from build123d import *

# Parameters (mm, degrees)
F1_DEPTH = 25
F2_DEPTH = 5
F3_R     = 5
F5_DEPTH = 1
F6_DEPTH = 5
F8_DEPTH = 1
F9_DEPTH = 5


with BuildPart() as f1:
    # F0 (on Right) → F1 (new body)
    with BuildSketch(Plane.YZ):
        Polygon((-1.9545168432, 38.6489601963), (-33.5964987424, 14.1788767986), (-28.2257758369, -25.4589250511), (-8.406874912, -22.7735635983), (-0.7535947717, -79.2574312341), (4.2011304595, -78.5860908709), (-3.9713255886, -18.2705245759), (3.1545996335, -0.8816359607), (10.2805248557, 16.5072526545), (58.4291094867, 53.742590351), (55.370349062, 57.6978380884), (10.2805248557, 22.8279692467), align=None)
        Polygon((-25.8654488138, -5.6400241263), (-7.3142972833, -13.2422419285), (-9.1963342424, -17.8348428934), (-23.9423909688, -19.8328594567), align=None, mode=Mode.SUBTRACT)
        Polygon((1.5615552233, 8.4168698067), (-1.4719884671, 1.0143288458), (-4.5055321574, -6.3882121151), (-5.26391808, -8.2388473554), (-11.7411414209, -5.5844966263), (-17.2930471416, -3.3093388585), (-23.7702704824, -0.6549881294), (-23.0118845598, 1.1956471108), (-16.944797179, 16.0007290327), (-16.1864112564, 17.851364273), (-9.7091879156, 15.1970135439), (-4.1572821949, 12.9218557761), (2.3199411459, 10.267505047), align=None, mode=Mode.SUBTRACT)
        Polygon((-14.6534166938, 22.50764705), (-2.8510041559, 31.6349520341), (6.2523573083, 19.863500585), (4.1741345282, 14.7921613112), align=None, mode=Mode.SUBTRACT)
        Polygon((-11.7411414209, -5.5844966263), (-10.9827554983, -3.7338613861), (-16.534661219, -1.4587036183), (-17.2930471416, -3.3093388585), align=None)
        Polygon((-10.4675738382, 13.3463783036), (-4.9156681175, 11.0712205358), (-4.1572821949, 12.9218557761), (-9.7091879156, 15.1970135439), align=None)
    extrude(amount=F1_DEPTH)

    # F0 (on Right) → F2 (join)
    with BuildSketch(Plane.YZ):
        Polygon((-5.26391808, -8.2388473554), (-4.5055321574, -6.3882121151), (-10.9827554983, -3.7338613861), (-11.7411414209, -5.5844966263), align=None)
        Polygon((-17.2930471416, -3.3093388585), (-16.534661219, -1.4587036183), (-23.0118845598, 1.1956471108), (-23.7702704824, -0.6549881294), align=None)
        Polygon((-16.944797179, 16.0007290327), (-10.4675738382, 13.3463783036), (-9.7091879156, 15.1970135439), (-16.1864112564, 17.851364273), align=None)
        Polygon((-4.9156681175, 11.0712205358), (1.5615552233, 8.4168698067), (2.3199411459, 10.267505047), (-4.1572821949, 12.9218557761), align=None)
    extrude(amount=F2_DEPTH)

    # F3
    f3_edges = [f1.edges().sort_by_distance(p)[0] for p in [
        (12.5, -33.596499, 14.178877),
    ]]
    fillet(f3_edges, radius=F3_R)

    # F4 (on face) → F5 (join)
    with BuildSketch(Plane(origin=(0, -7.1996627103, 9.3098006026), x_dir=(1, 0, 0), z_dir=(0, -0.6117520849, 0.7910495475))):
        with BuildLine():
            ThreePointArc((14, 56.8474623166), (16, 54.8474623166), (18, 56.8474623166))
            ThreePointArc((18, 56.8474623166), (16, 58.8474623166), (14, 56.8474623166))
        make_face()
        with BuildLine():
            ThreePointArc((14, 44.3474623166), (16, 42.3474623166), (18, 44.3474623166))
            ThreePointArc((18, 44.3474623166), (16, 46.3474623166), (14, 44.3474623166))
        make_face()
        with BuildLine():
            Line((18, 44.3474623166), (18, 56.8474623166))
            ThreePointArc((18, 56.8474623166), (16, 54.8474623166), (14, 56.8474623166))
            Line((14, 56.8474623166), (14, 44.3474623166))
            ThreePointArc((14, 44.3474623166), (16, 46.3474623166), (18, 44.3474623166))
        make_face()
    extrude(amount=F5_DEPTH)

    # F4 (on face) → F6 (cut)
    with BuildSketch(Plane(origin=(0, -7.1996627103, 9.3098006026), x_dir=(1, 0, 0), z_dir=(0, -0.6117520849, 0.7910495475))):
        with BuildLine():
            ThreePointArc((14, 64.8474623166), (16, 62.8474623166), (18, 64.8474623166))
            ThreePointArc((18, 64.8474623166), (16, 66.8474623166), (14, 64.8474623166))
        make_face()
        with BuildLine():
            ThreePointArc((14, 36.3474623166), (16, 34.3474623166), (18, 36.3474623166))
            ThreePointArc((18, 36.3474623166), (16, 38.3474623166), (14, 36.3474623166))
        make_face()
    extrude(amount=-F6_DEPTH, mode=Mode.SUBTRACT)

    # F7 (on face) → F8 (join)
    with BuildSketch(Plane(origin=(0, -11.2853910764, -1.5291137632), x_dir=(1, 0, 0), z_dir=(0, -0.9909450462, -0.1342680726))):
        with BuildLine():
            ThreePointArc((14, -43.6885751417), (16, -45.6885751417), (18, -43.6885751417))
            ThreePointArc((18, -43.6885751417), (16, -41.6885751417), (14, -43.6885751417))
        make_face()
        with BuildLine():
            Line((18, -56.1885751417), (18, -43.6885751417))
            ThreePointArc((18, -43.6885751417), (16, -45.6885751417), (14, -43.6885751417))
            Line((14, -43.6885751417), (14, -56.1885751417))
            ThreePointArc((14, -56.1885751417), (16, -54.1885751417), (18, -56.1885751417))
        make_face()
        with BuildLine():
            ThreePointArc((14, -56.1885751417), (16, -58.1885751417), (18, -56.1885751417))
            ThreePointArc((18, -56.1885751417), (16, -54.1885751417), (14, -56.1885751417))
        make_face()
    extrude(amount=F8_DEPTH)

    # F7 (on face) → F9 (cut)
    with BuildSketch(Plane(origin=(0, -11.2853910764, -1.5291137632), x_dir=(1, 0, 0), z_dir=(0, -0.9909450462, -0.1342680726))):
        with BuildLine():
            ThreePointArc((14, -35.6885751417), (16, -37.6885751417), (18, -35.6885751417))
            ThreePointArc((18, -35.6885751417), (16, -33.6885751417), (14, -35.6885751417))
        make_face()
        with BuildLine():
            ThreePointArc((14, -64.1885751417), (16, -66.1885751417), (18, -64.1885751417))
            ThreePointArc((18, -64.1885751417), (16, -62.1885751417), (14, -64.1885751417))
        make_face()
    extrude(amount=-F9_DEPTH, mode=Mode.SUBTRACT)


solid = f1.part
The model under review builds one solid part; all positions refer to its coordinate system, in mm. A direction names the side the tool comes from. Round coordinates to 2 decimals unless told otherwise and drop trailing zeros. Order: outer loops, then holes, each group sorted by start corner. A loop starts at its lowest first (then second) coordinate and runs counter-clockwise, first axis right, second up. Notation, with made-up numbers: (86, 6) -> (135, 6) arc R34 cw to (135, 44) -> close; hole circle Ø4 at (-11, -16.75). An arc over 180 degrees is marked (long way). Use CSV: the item, a comma, the result in double quotes. Start each with the question number.
(1) Consider section A-A on y = -19. Write out the cut boundary in (x, z), and give its area (3 significant figures).
(2) Consider section B-B on x = 20.75. State how many separate pieces and enclosed holes the cut face has, and give its area (3 significant figures).
(3) Mouldability with a two-part tool opening along Z and no side actions: class faces 1 (the face through (0, -1, 0)), 2 (the face through (14, -4.1, -36.5)), 3 (the face through (12.325, 4.249, 30.628)) as pulls with the +Z half, pulls with the -Z half, needs draft (parallel to the pull), parting line crosses it, or undercut.
(4) Wall thickness on probe 1 along Z at (x, y) = (5.75, -9); probe 2 along Z at (x, y) = (10.5, -14.5); probe 3 along Y at (x, z) = (16.25, 30.5): over which ranges is each line inside the solid? List them lowest first. Write a range as from..to.
(5) Tool access review of faces 4 (the face through (18, 32.5, 40.6)), 5 (the face through (18, -5, -51)), 6 (the face through (12.325, -18.455, -24.135)), 7 (the face through (14.86, -20.49, -2)): name each direction out of +Z, -Z, +X, -X, +Y, -Y from which nothing blocks a thin tool from reaching the whole face with its end or side.
(6) Consider section C-C on y = 34. Write out the cut boundary in (x, z).
(7) Insertion check: pin 1 (5 mm diameter, centred on x = 18, z = -26.5, fed in from +Y); pin 2 (3.5 mm diameter, centred on y = -7, z = -5, fed in from +X); pin 3 (8 mm diameter, centred on x = 15, z = -38, fed in from +Y). Each pin has a flat end and moves straight along its axis. Give the tip position at first contact, or say it passes through.
(8) Consider section D-D on y = 18.5. Write out the cut boundary in (x, z), and give its area (3 significant figures).
Responses:
1,outline,"(0, -24.21) -> (25, -24.21) -> (25, -19.16) -> (0, -19.16) -> close; (0, -8.45) -> (25, -8.45) -> (25, -2.61) -> (5, -2.61) -> (5, -0.45) -> (0, -0.45) -> close; (0, 10.99) -> (25, 10.99) -> (25, 25.47) -> (0, 25.47) -> close"
1,area,"645 mm²"
2,separate pieces,"1"
2,enclosed holes,"3"
2,area,"1,710 mm²"
3,face 1,"needs draft"
3,face 2,"undercut"
3,face 3,"pulls with the +Z half"
4,probe 1,"-22.85..-17.36, -12.55..-6.71, 12.74..20.19, 26.88..33.2"
4,probe 2,"-23.6..-18.55, -10.3..-2.29, 17.16..22.44, 22.63..28.95"
4,probe 3,"-12.49..-4.32, -1.97..4.35, 24.87..28.37"
5,face 4,"+Z, +X"
5,face 5,"-Z, +X, -Y"
5,face 6,"-Z, +X, -X"
5,face 7,"+X"
6,outline,"(0, 34.85) -> (25, 34.85) -> (25, 41.17) -> (18, 41.17) -> (18, 42.44) -> (14, 42.44) -> (14, 41.17) -> (0, 41.17) -> close"
7,pin 1,"y = -2.52"
7,pin 2,"x = 5"
7,pin 3,"y = -0.76"
8,outline,"(0, 22.86) -> (25, 22.86) -> (25, 29.18) -> (0, 29.18) -> close"
8,area,"158 mm²"
